```python
from build123d import *

# Parameters (mm, degrees)
SKETCH1_W           = 7
SKETCH1_H           = 10
BOSS_EXTRUDE1_DEPTH = 76.2
SKETCH6_R           = 2
CUT_EXTRUDE3_DEPTH  = 13


with BuildPart() as part:
    # Sketch1 → Boss-Extrude1 (new, symmetric)
    with BuildSketch(Plane(origin=(0, 0, 0), x_dir=(1, 0, 0), z_dir=(0, 1, 0))):
        Rectangle(SKETCH1_W, SKETCH1_H)
    extrude(amount=BOSS_EXTRUDE1_DEPTH, both=True)

    # Sketch6 → Cut-Extrude3 (cut)
    with BuildSketch(Plane.XZ.offset(76.2)):
        with Locations(Location((0, 0, 0), (0, 0, 270))):
            Circle(SKETCH6_R)
    cut_extrude3 = extrude(amount=-CUT_EXTRUDE3_DEPTH, mode=Mode.SUBTRACT)

    # Mirror1: Cut-Extrude3 across plane
    add(cut_extrude3.mirror(Plane.ZX), mode=Mode.SUBTRACT)


solid = part.part
```
CAD build for the part. Positions are in the model's coordinates, mm. A direction names the side the tool comes from. Round coordinates to 2 decimals unless told otherwise and drop trailing zeros. Write each loop counter-clockwise with the first axis right and the second up, starting at its lowest first coordinate (ties: lowest second). Pieces come first, ordered by that corner, then holes. Notation, with made-up numbers: (-39.75, 21.5) - (-18.75, 21.5) arc R19 cw to (-18.75, 38.5) - close; hole circle Ø2 at (67, 79.25). An arc over 180 degrees is marked (long way). Return JSON: item names as keys, results as strings. Group by question number.
Item 1: Mould opens along X. For faces 1 (the face through (3.5, 1, 0)), 2 (the face through (0, 1, -5)), 3 (the face through (-2, -70, 0)), 4 (the face through (0, -63.2, 0)) say: +X half, -X half, draft (parallel to the pull), parting line (faces both ways), or undercut.
Item 2: Flat gauge pins, fed straight in: pin 1 Ø3 at (x, z) = (0, 0) entering from +Y; pin 2 Ø1.2 at (x, z) = (1, -0.5) entering from -Y. Where does each tip first touch, or does it go through?
Item 3: Band-saw the part on B-B on z = 0. List the corners of the cut face in (x, y), plus the area to 3 significant figures.
Item 4: 3-axis set-ups, long thin cutter, end or side, ignore diameter. For faces 5 (the face through (0, 76.2, -2.3)), 6 (the face through (-2, 70, 0)): which of +Z, -Z, +X, -X, +Y, -Y reach the whole face in a straight line?
Item 5: Probe probe 1 along X at (y, z) = (-67, 0); probe 2 along Y at (x, z) = (1, 0.5); probe 3 along Z at (x, y) = (-1, 69). List the from-to ranges inside material, lowest first.
Item 6: Band-saw the part on A-A on x = 0. List the corners of the cut face in (y, z), plus the area to 3 significant figures.
Resolved:
{
 "1": {"face 1": "+X half", "face 2": "draft", "face 3": "undercut", "face 4": "undercut"},
 "2": {"pin 1": "stops at y = 63.2", "pin 2": "stops at y = -63.2"},
 "3": {"outline": "(-3.5, -76.2) - (-2, -76.2) - (-2, -63.2) - (2, -63.2) - (2, -76.2) - (3.5, -76.2) - (3.5, 76.2) - (2, 76.2) - (2, 63.2) - (-2, 63.2) - (-2, 76.2) - (-3.5, 76.2) - close", "area": "963 mm²"},
 "4": {"face 5": "+Z, -Z, +X, -X, +Y", "face 6": "+Y"},
 "5": {"probe 1": "x = -3.5 to -2, 2 to 3.5", "probe 2": "y = -63.2 to 63.2", "probe 3": "z = -5 to -1.73, 1.73 to 5"},
 "6": {"outline": "(-76.2, -5) - (76.2, -5) - (76.2, -2) - (63.2, -2) - (63.2, 2) - (76.2, 2) - (76.2, 5) - (-76.2, 5) - (-76.2, 2) - (-63.2, 2) - (-63.2, -2) - (-76.2, -2) - close", "area": "1,420 mm²"}
}
